Geometry check sheet. Reference: the model listing, model coordinates, mm. Face numbers are marked on the shaded views. A direction names the side the tool comes from. Round coordinates to 2 decimals unless told otherwise and drop trailing zeros. Write each loop counter-clockwise with the first axis right and the second up, starting at its lowest first coordinate (ties: lowest second). Pieces come first, ordered by that corner, then holes. Notation, with made-up numbers: M -27,11 L 25,11 A22 ccw 25,37 Z; hole C -30,-1 d10. An arc over 180 degrees is marked long. Use a Markdown table: item, result.
```python
from build123d import *

# Parameters (mm, degrees)
SKETCH1_R           = 3
BOSS_EXTRUDE1_DEPTH = 2
BOSS_EXTRUDE2_DEPTH = 2
CUT_EXTRUDE1_DEPTH  = 2
BOSS_EXTRUDE3_DEPTH = 3
CUT_EXTRUDE2_DEPTH  = 13


with BuildPart() as part:
    # Sketch1 → Boss-Extrude1 (new body)
    with BuildSketch(Plane(origin=(0, 0, 0), x_dir=(1, 0, 0), z_dir=(0, 1, 0))):
        with BuildLine():
            Line((9, 4), (9, 6))
            Line((9, 6), (-9, 6))
            ThreePointArc((-9, 6), (-15, 0), (-9, -6))
            Line((-9, -6), (9, -6))
            Line((9, -6), (9, -4))
            Line((9, -4), (6, -4))
            Line((6, -4), (6, 4))
            Line((6, 4), (9, 4))
        make_face()
        with Locations((-9, 0)):
            Circle(SKETCH1_R, mode=Mode.SUBTRACT)
    extrude(amount=BOSS_EXTRUDE1_DEPTH)

    # Sketch2 → Boss-Extrude2 (add)
    with BuildSketch(Plane(origin=(0, 2, 0), x_dir=(1, 0, 0), z_dir=(0, 1, 0))):
        Polygon((9, 6), (-1.205687829, 6), (-1.205687829, 4), (-4.205687829, 4), (-4.205687829, -4), (-1.205687829, -4), (-1.205687829, -6), (9, -6), (9, -4), (6, -4), (6, 4), (9, 4), align=None)
    extrude(amount=BOSS_EXTRUDE2_DEPTH)

    # Sketch3 → Cut-Extrude1 (cut, symmetric)
    with BuildSketch(Plane.XY):
        Polygon((-1.205687829, 4), (-4.205687829, 2), (-4.205687829, 4), align=None)
    extrude(amount=CUT_EXTRUDE1_DEPTH, both=True, mode=Mode.SUBTRACT)

    # Sketch4 → Boss-Extrude3 (add)
    with BuildSketch(Plane(origin=(0, 4, 0), x_dir=(1, 0, 0), z_dir=(0, 1, 0))):
        Polygon((9, 6), (-1.205687829, 6), (-1.205687829, 4), (1.794312171, 2), (1.794312171, -2), (-1.205687829, -4), (-1.205687829, -6), (9, -6), (9, -4), (6, -4), (6, 4), (9, 4), align=None)
    extrude(amount=BOSS_EXTRUDE3_DEPTH)

    # Sketch5 → Cut-Extrude2 (cut)
    with BuildSketch(Plane(origin=(6, 0, 0), x_dir=(0, 0, -1), z_dir=(1, 0, 0))):
        Polygon((2, 7), (2, 6), (-2, 7), align=None)
    extrude(amount=-CUT_EXTRUDE2_DEPTH, mode=Mode.SUBTRACT)


solid = part.part
```
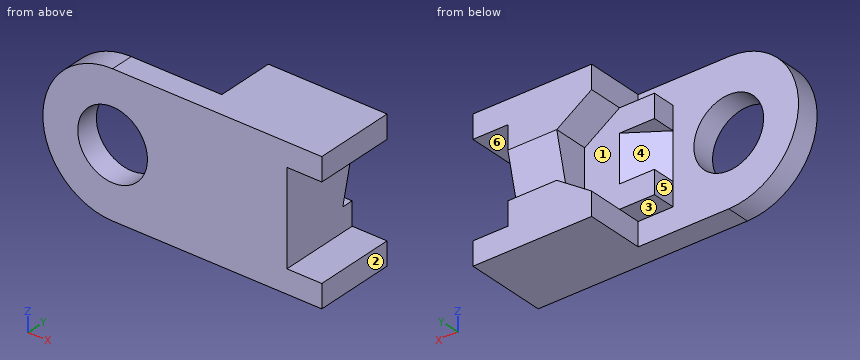
Item 1: Material ranges on line 1 along X through (y, z) = (1.4, 0); line 2 along Z through (x, y) = (-9, 1.15); line 3 along Z through (x, y) = (6.5, 2.25), recorded low to high. Write a range as from..to.
Outcome:
| item | result |
|---|---|
| line 1 | x = -15..-12, -6..6 |
| line 2 | z = -6..-3, 3..6 |
| line 3 | z = -6..-4, 4..6 |
Item 2: Go/stop test with flat-tipped pins: pin 1 (4 mm diameter, centred on x = -6, z = 1, fed in from +Y); pin 2 (1 mm diameter, centred on x = -2.5, y = 3, fed in from -Z); pin 3 (1.6 mm diameter, centred on x = -3, y = 3, fed in from +Z). Record where each tip stops, or that it passes through.
Outcome:
| item | result |
|---|---|
| pin 1 | stops at y = 2.14 |
| pin 2 | stops at z = -4 |
| pin 3 | stops at z = 4 |
Item 3: Cross-section at A-A, the plane z = 0. Record the cut outline in (x, y), and give its area (3 significant figures).
Outcome:
| item | result |
|---|---|
| outline | M -15,0 L -12,0 L -12,2 L -15,2 Z; M -6,0 L 6,0 L 6,6.5 L 1.79,6.5 L 1.79,4 L -1.21,4 L -4.21,2 L -6,2 Z |
| area | 57.9 mm2 |
Item 4: Mould release check, pull along Z, two halves, no side actions. Record for the marked faces 1, 2 and 3: +Z half, -Z half, draft (parallel to the pull), parting line (faces both ways), or undercut.
Outcome:
| item | result |
|---|---|
| face 1 | undercut |
| face 2 | draft |
| face 3 | -Z half |
Item 5: Cross-section at D-D, the plane y = 5.75. Record the cut outline in (x, z), and give its area (3 significant figures).
Outcome:
| item | result |
|---|---|
| outline | M -1.21,-6 L 9,-6 L 9,-4 L 6,-4 L 6,4 L 9,4 L 9,6 L -1.21,6 L -1.21,4 L 1.79,2 L 1.79,-2 L -1.21,-4 Z |
| area | 80.5 mm2 |
Item 6: Cross-section at B-B, the plane y = 0.75. Record the cut outline in (x, z).
Outcome:
| item | result |
|---|---|
| outline | M -9,-6 L 9,-6 L 9,-4 L 6,-4 L 6,4 L 9,4 L 9,6 L -9,6 A6 ccw Z; hole C -9,0 d6 |
Item 7: Access from +Z, -Z, +X, -X, +Y, -Y to the whole of each face (thin tool, end or side, straight path). Record for the marked faces 4, 5 and 6.
Outcome:
| item | result |
|---|---|
| face 4 | -X, +Y |
| face 5 | +Z, -Z, -X, +Y |
| face 6 | +X, +Y, -Y |
Item 8: Cross-section at C-C, the plane x = 4. Record the cut outline in (y, z).
Outcome:
| item | result |
|---|---|
| outline | M 0,-6 L 7,-6 L 7,-2 L 6,-2 L 7,2 L 7,6 L 0,6 Z |
